Check sheet for the modelled part. Datum: model origin and axes. Units: mm. Face numbers are marked on the shaded views. A direction names the side the tool comes from. Round coordinates to 2 decimals unless told otherwise and drop trailing zeros. Write each loop counter-clockwise with the first axis right and the second up, starting at its lowest first coordinate (ties: lowest second). Pieces come first, ordered by that corner, then holes. Notation, with made-up numbers: (17.25, 17.5) - (64.25, 17.5) arc R32 cw to (64.25, 43.5) - close; hole circle Ø10 at (-20, 17). An arc over 180 degrees is marked (long way). Use one line per item in the form item = value. Start each with the question number.
1) Section check C-C (z = 1.5). Record the boundary of the cut face in (x, y), then the cut area to 3 significant figures.
2) Section check B-B (x = 0). Record the boundary of the cut face in (y, z).
3) Draft check along Y on the marked faces 1, 2 and 3. Enter one of: +Y half, -Y half, draft (parallel to the pull), parting line (faces both ways), or undercut.
4) Scan lines: probe 1 along Y at (x, z) = (0, 2.15); probe 2 along Y at (x, z) = (3, -1.25); probe 3 along Z at (x, y) = (3, -12.75). Record each from-to range of solid material in increasing order.
5) Set-up check for the marked faces 4, 5 and 6: record each of +Z, -Z, +X, -X, +Y, -Y from which the full face is reachable in a straight line by a thin tool's end or side.
6) Section check D-D (y = -10.75). Record the boundary of the cut face in (x, z), then the cut area to 3 significant figures.
7) Section check A-A (y = 11.5). Record the boundary of the cut face in (x, z), then the cut area to 3 significant figures.
8) Gauge pin test, flat ends, axial feed: P1, Ø1.6, axis at x = -1.5, z = -1, coming from the +Y side; P2, Ø2, axis at x = 1.5, y = -10.5, coming from the +Z side; P3, Ø3.5, axis at x = 0, y = 11.5, coming from the -Z side. Record the tip position at first contact, or that the pin passes through.
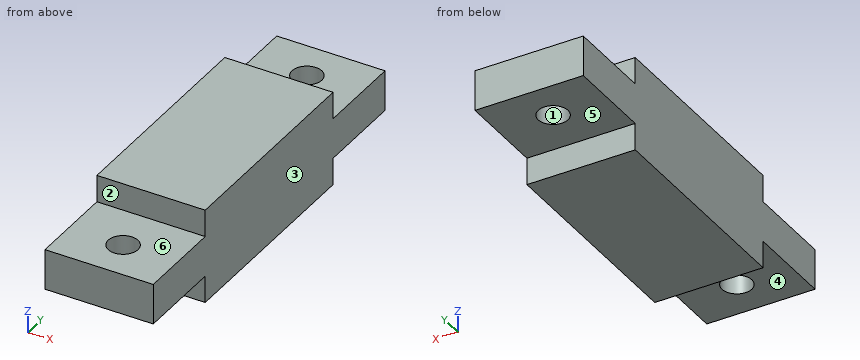
from build123d import *

# Parameters (mm, degrees)
SKETCH_1_W            = 8
SKETCH_1_H            = 29
EXTRUDE_272_DEPTH     = 3
SKETCH_2_W            = 8
SKETCH_2_H            = 16
EXTRUDE_392_DEPTH     = 2
EXTRUDE_START         = 3
SKETCH_2_2_W          = 8
SKETCH_2_2_H          = 16
EXTRUDE_443_DEPTH     = 2
CUT_EXTRUDE_679_REACH = 17.851
SKETCH_3_R            = 1.1


with BuildPart() as part:
    # 草图1 → Extrude 272 (new body)
    with BuildSketch(Plane.XY):
        Rectangle(SKETCH_1_W, SKETCH_1_H)
    extrude(amount=EXTRUDE_272_DEPTH)

    # 草图2 → Extrude 392 (add)
    with BuildSketch(Plane.XY):
        Rectangle(SKETCH_2_W, SKETCH_2_H)
    extrude(amount=-EXTRUDE_392_DEPTH)

    # 草图2<2> → Extrude 443 (add)
    with BuildSketch(Plane.XY.offset(EXTRUDE_START)):
        Rectangle(SKETCH_2_2_W, SKETCH_2_2_H)
    extrude(amount=EXTRUDE_443_DEPTH)

    # 草图3 → Cut-Extrude 679 (cut, up to next)
    with BuildSketch(Plane.XY.offset(3), mode=Mode.PRIVATE) as cut_extrude_679_sk1:
        with Locations((0, 11.5)):
            Circle(SKETCH_3_R)
    cut_extrude_679_tool1 = extrude(cut_extrude_679_sk1.sketch, amount=-CUT_EXTRUDE_679_REACH, mode=Mode.PRIVATE) & part.part
    # 草图3 → Cut-Extrude 679 (cut, up to next)
    with BuildSketch(Plane.XY.offset(3), mode=Mode.PRIVATE) as cut_extrude_679_sk2:
        with Locations((0, -11.5)):
            Circle(SKETCH_3_R)
    cut_extrude_679_tool2 = extrude(cut_extrude_679_sk2.sketch, amount=-CUT_EXTRUDE_679_REACH, mode=Mode.PRIVATE) & part.part
    add(cut_extrude_679_tool1.solids().sort_by_distance((0, 11.5, 3))[0], mode=Mode.SUBTRACT)
    add(cut_extrude_679_tool2.solids().sort_by_distance((0, -11.5, 3))[0], mode=Mode.SUBTRACT)


solid = part.part
Results are:
q1.outline = (-4, -14.5) - (4, -14.5) - (4, 14.5) - (-4, 14.5) - close; hole circle Ø2.2 at (0, -11.5); hole circle Ø2.2 at (0, 11.5)
q1.area = 224 mm²
q2.outline = (-14.5, 0) - (-12.6, 0) - (-12.6, 3) - (-14.5, 3) - close; (-10.4, 0) - (-8, 0) - (-8, -2) - (8, -2) - (8, 0) - (10.4, 0) - (10.4, 3) - (8, 3) - (8, 5) - (-8, 5) - (-8, 3) - (-10.4, 3) - close; (12.6, 0) - (14.5, 0) - (14.5, 3) - (12.6, 3) - close
q3.face_1 = undercut
q3.face_2 = -Y half
q3.face_3 = draft
q4.probe_1 = -14.5 to -12.6, -10.4 to 10.4, 12.6 to 14.5
q4.probe_2 = -8 to 8
q4.probe_3 = 0 to 3
q5.face_4 = -Z, +X, -X, -Y
q5.face_5 = -Z, +X, -X, +Y
q5.face_6 = +Z, +X, -X, -Y
q6.outline = (-4, 0) - (-0.8, 0) - (-0.8, 3) - (-4, 3) - close; (0.8, 0) - (4, 0) - (4, 3) - (0.8, 3) - close
q6.area = 19.2 mm²
q7.outline = (-4, 0) - (-1.1, 0) - (-1.1, 3) - (-4, 3) - close; (1.1, 0) - (4, 0) - (4, 3) - (1.1, 3) - close
q7.area = 17.4 mm²
q8.P1 = 8
q8.P2 = 3
q8.P3 = 0
